Part model, mm, in its own coordinate system. Coordinates: 2 decimals unless noted, no trailing zeros. Order: outer loops, then holes, each group sorted by start corner. A loop starts at its lowest first (then second) coordinate and runs counter-clockwise, first axis right, second up.
from build123d import *

# Parameters (mm, degrees)
F2_DEPTH = 5
F3_DEPTH = 1.2
F4_R     = 0.4
F5_DEPTH = 2.5
F6_R     = 0.4
F7_DEPTH = 5
F8_R     = 2.49999
F9_R     = 2.5


# Not quite as in the source:
# - a fillet or chamfer is up to 0.001 mm smaller than in the source, because OpenCascade refuses the exact size


with BuildPart() as f2:
    # F1 (on Top) → F2 (new body)
    with BuildSketch(Plane.XY):
        Polygon((-60, -46.1892857143), (-0.7, -46.1892857143), (60, -46.1892857143), (60, 60.5107142857), (0, 60.5107142857), (-60, 60.5107142857), align=None)
        Polygon((-27.75, -16.6892857143), (0, -16.6892857143), (27.75, -16.6892857143), (27.75, -36.3892857143), (-0.7, -36.3892857143), (-27.75, -36.3892857143), align=None, mode=Mode.SUBTRACT)
        Polygon((27.75, -16.6892857143), (0, -16.6892857143), (-27.75, -16.6892857143), (-27.75, -36.3892857143), (-0.7, -36.3892857143), (27.75, -36.3892857143), align=None)
    extrude(amount=-F2_DEPTH)

    # F1 (on Top) → F3 (cut)
    with BuildSketch(Plane.XY):
        Polygon((27.75, -16.6892857143), (0, -16.6892857143), (-27.75, -16.6892857143), (-27.75, -36.3892857143), (-0.7, -36.3892857143), (27.75, -36.3892857143), align=None)
    extrude(amount=-F3_DEPTH, mode=Mode.SUBTRACT)

    # F4 (on face) → F5 (cut, symmetric)
    with BuildSketch(Plane(origin=(-60, 0, 0), x_dir=(0, -1, 0), z_dir=(-1, 0, 0))):
        with Locations((-58.0107142857, -2.5)):
            Circle(F4_R)
    extrude(amount=F5_DEPTH, both=True, mode=Mode.SUBTRACT)

    # F6 (on face) → F7 (cut)
    with BuildSketch(Plane.YZ.offset(60)):
        with Locations((58.0107142857, -2.5)):
            Circle(F6_R)
    extrude(amount=-F7_DEPTH, mode=Mode.SUBTRACT)

    # F8 (radius 2.5 in the source; OpenCascade refuses exactly that, so slightly less here)
    f8_edges = [f2.edges().sort_by_distance(p)[0] for p in [
        (0, 60.510714, 0),
        (0, 60.510714, -5),
    ]]
    fillet(f8_edges, radius=F8_R)

    # F9
    f9_edges = [f2.edges().sort_by_distance(p)[0] for p in [
        (0, -46.189286, -5),
    ]]
    fillet(f9_edges, radius=F9_R)


solid = f2.part
Q1. Pin check, flat tips, straight feed: pin 1 Ø1.5 at (x, z) = (-11, -3.5) entering from -Y; pin 2 Ø6 at (x, y) = (3, -26.5) entering from +Z; pin 3 Ø0.6 at (x, z) = (-6.5, -0.5) entering from +Y. Stop position of each tip, or through.
Results list:
pin 1: stops at y = -46.18
pin 2: stops at z = -1.2
pin 3: stops at y = 59.84
Q2. Cut at A-A on y = -33.5. Write the cut outline in (x, z).
Results list:
outline: (-60, -5) - (60, -5) - (60, 0) - (27.75, 0) - (27.75, -1.2) - (-27.75, -1.2) - (-27.75, 0) - (-60, 0) - close
Q3. Mould opens along X. For faces 1 (the face through (0.84, -45.438, -4.287)), 2 (the face through (-60, 8, -2)), 3 (the face through (0, -26, -1.2)) say: pulls with the +X half, pulls with the -X half, needs draft (parallel to the pull), parting line crosses it, or undercut.
Results list:
face 1: needs draft
face 2: pulls with the -X half
face 3: undercut
Q4. Wall check: line 1 along Y through (x, z) = (30.5, -2.8); line 2 along Y through (x, z) = (-51.5, -3.45). Give the ranges that are in metal, low to high.
Results list:
line 1: y = -46.17 to 60.49
line 2: y = -46 to 60.32
